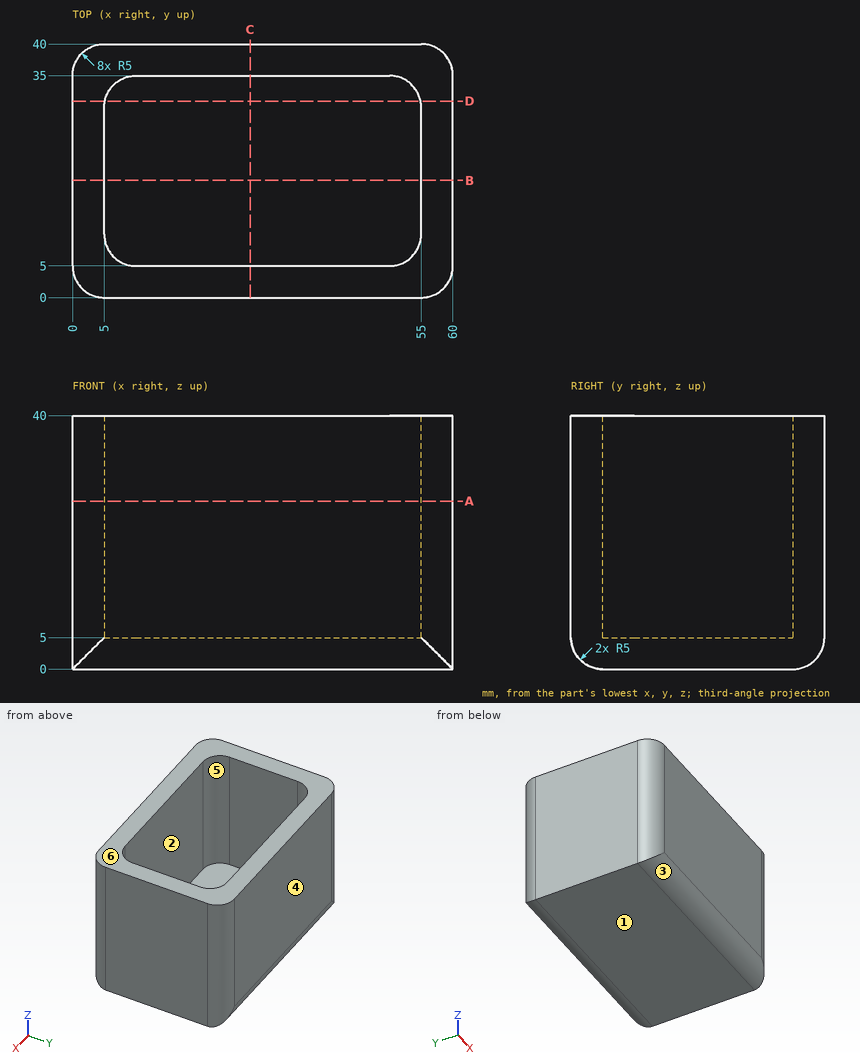
Source: three-view drawing plus pictorial views. Frame: mm from the lowest corner of the part. A direction names the side the tool comes from. Round coordinates to 2 decimals unless told otherwise and drop trailing zeros. Write each loop counter-clockwise with the first axis right and the second up, starting at its lowest first coordinate (ties: lowest second). Pieces come first, ordered by that corner, then holes. Notation, with made-up numbers: M -33.5,-4.75 L -26.5,-4.75 A34 cw -26.5,30.25 Z; hole C -25.5,63 d11. An arc over 180 degrees is marked long. One line per item, written item: value. Start each with the question number.
Item 1: Section query B-B (y = 18.5). Return the cut outline in (x, z), plus the area to 3 significant figures.
Item 2: Section query D-D (y = 31). Return the cut outline in (x, z), plus the area to 3 significant figures.
Item 3: Mould query, pull axis Y, two halves, no side actions, for the marked faces 3, 4, 5 and 6. Classes: pulls with the +Y half, pulls with the -Y half, needs draft (parallel to the pull), parting line crosses it, or undercut.
Item 4: Section query C-C (x = 28). Return the cut outline in (y, z), plus the area to 3 significant figures.
Item 5: Pin query (flat end, axial travel): pin 1 (9 mm diameter, centred on x = 34, y = 19.5, fed in from +Z). Return the tip coordinate at first contact, or that it passes through.
Item 6: Ray query, L1, parallel to Y at x = 49, z = 26.5; L2, parallel to X at y = 19, z = 12; L3, parallel to Z at x = 23, y = 16. Return the intervals inside material, ascending. Write a range as from..to.
Item 7: Section query A-A (z = 26.5). Return the cut outline in (x, y).
Item 8: Set-up query: the marked faces 1 and 2. Return all of +Z, -Z, +X, -X, +Y, -Y with unobstructed straight access to the full face (end or side cutting, diameter ignored); none if empty.
Result set:
1. outline: M 0,0 L 60,0 L 60,40 L 55,40 L 55,5 L 5,5 L 5,40 L 0,40 Z
1. area: 650 mm²
2. outline: M 0,0 L 60,0 L 60,40 L 54.9,40 L 54.9,5 L 5.1,5 L 5.1,40 L 0,40 Z
2. area: 657 mm²
3. face 3: pulls with the -Y half
3. face 4: pulls with the +Y half
3. face 5: undercut
3. face 6: needs draft
4. outline: M 0,5 A5 ccw 5,0 L 35,0 A5 ccw 40,5 L 40,40 L 35,40 L 35,5 L 5,5 L 5,40 L 0,40 Z
4. area: 539 mm²
5. pin 1: stops at z = 5
6. L1: y = 0..5, 35..40
6. L2: x = 0..5, 55..60
6. L3: z = 0..5
7. outline: M 0,5 A5 ccw 5,0 L 55,0 A5 ccw 60,5 L 60,35 A5 ccw 55,40 L 5,40 A5 ccw 0,35 Z; hole M 5,10 A5 ccw 10,5 L 50,5 A5 ccw 55,10 L 55,30 A5 ccw 50,35 L 10,35 A5 ccw 5,30 Z
8. face 1: -Z, +X, -X, +Y, -Y
8. face 2: +Z
